Geometry check sheet. Reference: drawing and pictorial views, mm from the part's lowest x, y, z. Give positions to 0.01 mm unless a question says otherwise; leave off trailing zeros. Write each loop counter-clockwise with the first axis right and the second up, starting at its lowest first coordinate (ties: lowest second). Pieces come first, ordered by that corner, then holes. Notation, with made-up numbers: M 46,71 L 90,71 A36 cw 90,106 Z; hole C 59.25,39.5 d10. An arc over 180 degrees is marked long. One line per item, written item: value. Start each with the question number.
1. Cross-section at C-C on y = 31. Record the cut outline in (x, z).
2. Cross-section at B-B on x = 96.5. Record the cut outline in (y, z).
3. Scan lines: line 1 (X direction, y = 81.5, z = 2.5) (1 decimal); line 2 (Y direction, x = 48.5, z = 2.3) (1 decimal); line 3 (X direction, y = 87.5, z = 1.75) (1 decimal). Record each from-to range of solid material in increasing order.
4. Cross-section at A-A on z = 0.7. Count the separate pieces of the cut face and the enclosed holes in it, then the cut area to 3 significant figures.
5. Gauge pin test, flat end, axial feed: pin 1 (1 mm diameter, centred on x = 36, y = 40, fed in from +Z). Record the tip position at first contact, or that the pin passes through.
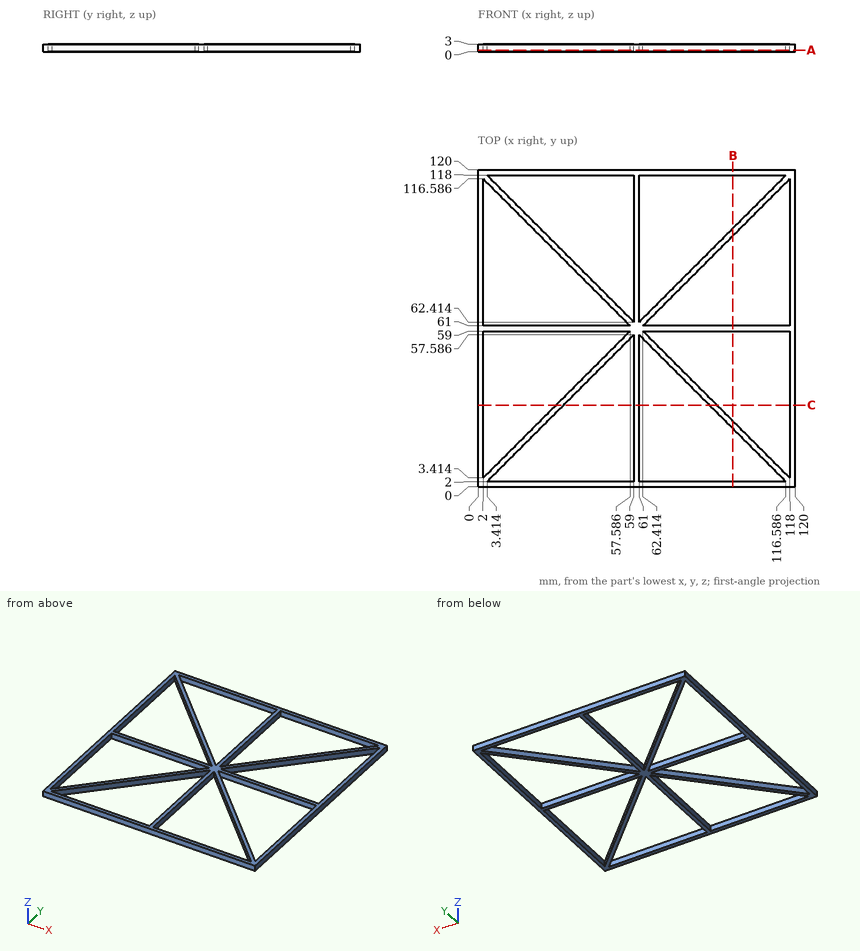
Report:
1. outline: M 0,0 L 2,0 L 2,3 L 0,3 Z; M 29.59,0 L 32.41,0 L 32.41,3 L 29.59,3 Z; M 59,0 L 61,0 L 61,3 L 59,3 Z; M 87.59,0 L 90.41,0 L 90.41,3 L 87.59,3 Z; M 118,0 L 120,0 L 120,3 L 118,3 Z
2. outline: M 0,0 L 2,0 L 2,3 L 0,3 Z; M 22.09,0 L 24.91,0 L 24.91,3 L 22.09,3 Z; M 59,0 L 61,0 L 61,3 L 59,3 Z; M 95.09,0 L 97.91,0 L 97.91,3 L 95.09,3 Z; M 118,0 L 120,0 L 120,3 L 118,3 Z
3. line 1: x = 0 to 2, 37.1 to 39.9, 59 to 61, 80.1 to 82.9, 118 to 120
3. line 2: y = 0 to 2, 47.1 to 49.9, 59 to 61, 70.1 to 72.9, 118 to 120
3. line 3: x = 0 to 2, 31.1 to 33.9, 59 to 61, 86.1 to 88.9, 118 to 120
4. separate pieces: 1
4. enclosed holes: 8
4. area: 2,040 mm^2
5. pin 1: passes through
